Here's how the part is built. I have some questions about the finished solid (model axes, mm). A direction names the side the tool comes from. Coordinates: 2 decimals unless noted, no trailing zeros. Order: outer loops, then holes, each group sorted by start corner. A loop starts at its lowest first (then second) coordinate and runs counter-clockwise, first axis right, second up.
```python
from build123d import *

# Parameters (mm, degrees)
SKETCH2_W           = 21.1
SKETCH2_H           = 50.65
SKETCH2_R           = 5.475
BOSS_EXTRUDE1_DEPTH = 7.5
SKETCH3_W           = 3.15
SKETCH3_H           = 10.4
CUT_EXTRUDE1_DEPTH  = 53.277863384
FILLET1_R           = 0.5
SKETCH4_W           = 11.1
SKETCH4_H           = 21
CUT_EXTRUDE3_DEPTH  = 13
SKETCH6_W           = 11.1
SKETCH6_H           = 18.940672382
CUT_EXTRUDE4_DEPTH  = 13
SKETCH7_W           = 11.1
SKETCH7_H           = 5
CUT_EXTRUDE5_DEPTH  = 1
SKETCH8_W           = 9
SKETCH8_H           = 3
CUT_EXTRUDE6_DEPTH  = 9.8


with BuildPart() as part:
    # Sketch2 → Boss-Extrude1 (new, symmetric)
    with BuildSketch(Plane.XY):
        with Locations((0, 6.8)):
            Rectangle(SKETCH2_W, SKETCH2_H)
        with Locations((0, 6.8)):
            Circle(SKETCH2_R, mode=Mode.SUBTRACT)
    extrude(amount=BOSS_EXTRUDE1_DEPTH, both=True)

    # Sketch3 → Cut-Extrude1 (cut, symmetric)
    with BuildSketch(Plane(origin=(0, 32.125, 0), x_dir=(1, 0, 0), z_dir=(0, 1, 0))):
        with Locations((-8.975, 0)):
            Rectangle(SKETCH3_W, SKETCH3_H)
    cut_extrude1 = extrude(amount=CUT_EXTRUDE1_DEPTH, both=True, mode=Mode.SUBTRACT)

    # Mirror1: Cut-Extrude1 across plane
    add(cut_extrude1.mirror(Plane(origin=(0, 0, 0), x_dir=(0, 0, 1), z_dir=(1, 0, 0))), mode=Mode.SUBTRACT)

    # Fillet1
    fillet1_edges = [part.edges().sort_by_distance(p)[0] for p in [
        (-7.4, 6.8, -5.2),
        (-7.4, 6.8, 5.2),
        (7.4, 6.8, 5.2),
        (7.4, 6.8, -5.2),
    ]]
    fillet(fillet1_edges, radius=FILLET1_R)

    # Sketch4 → Cut-Extrude3 (cut)
    with BuildSketch(Plane(origin=(0, 0, -7.5), x_dir=(-1, 0, 0), z_dir=(0, 0, -1))):
        with Locations((0, 11.825)):
            Rectangle(SKETCH4_W, SKETCH4_H)
    extrude(amount=-CUT_EXTRUDE3_DEPTH, mode=Mode.SUBTRACT)

    # Sketch6 → Cut-Extrude4 (cut)
    with BuildSketch(Plane(origin=(0, 0, -7.5), x_dir=(-1, 0, 0), z_dir=(0, 0, -1))):
        with Locations((0, -10.645336191)):
            Rectangle(SKETCH6_W, SKETCH6_H)
    extrude(amount=-CUT_EXTRUDE4_DEPTH, mode=Mode.SUBTRACT)

    # Sketch7 → Cut-Extrude5 (cut)
    with BuildSketch(Plane(origin=(0, 0, 5.5), x_dir=(-1, 0, 0), z_dir=(0, 0, -1))):
        with Locations((0, 19.825)):
            Rectangle(SKETCH7_W, SKETCH7_H)
    extrude(amount=-CUT_EXTRUDE5_DEPTH, mode=Mode.SUBTRACT)

    # Sketch8 → Cut-Extrude6 (cut)
    with BuildSketch(Plane(origin=(0, 32.125, 0), x_dir=(1, 0, 0), z_dir=(0, 1, 0))):
        with Locations((0, 4.5)):
            Rectangle(SKETCH8_W, SKETCH8_H)
    extrude(amount=-CUT_EXTRUDE6_DEPTH, mode=Mode.SUBTRACT)


solid = part.part
```
Q1. I need wall thicknesses on L1, parallel to Y at x = 4, z = 4 (3 decimals); L2, parallel to X at y = 6.8, z = 6.3 (3 decimals); L3, parallel to Y at x = 0, z = 7.05 (3 decimals). Which ranges of each line are inside material? Lowest first, please.
Q2. We'd pull the mould along Z, two halves only. Please class faces 5 (the flat face through (10.55, 6, 6)), 6 (the flat face through (-7, 13, -7.5)), 7 (the flat face through (7.4, 7, 0)), 8 (the flat face through (-9, 7, 5.2)): pulls with the +Z half, pulls with the -Z half, needs draft (parallel to the pull), parting line crosses it, or undercut.
Q3. If we section it at B-B on z = -1.25: Write out the boundary of the cut face in (x, y) (3 decimals).
Q4. For faces 1 (the flat face through (0, -1.175, -1)), 2 (the flat face through (-7.4, 7, 0)), 3 (the flat face through (5.55, 12, -1)), 4 (the flat face through (-4.5, 27, -4)), which set-ups out of +Z, -Z, +X, -X, +Y, -Y let a thin tool reach every point of the face, with its end or its side?
Q5. Will these pins go through, and if not, where does the flat tip stop? pin 1 (7.5 mm diameter, centred on y = -5.5, z = -0.5, fed in from +X); pin 2 (2 mm diameter, centred on y = 13.5, z = -3.5, fed in from -X); pin 3 (4 mm diameter, centred on x = -1.5, y = 19, fed in from -Z).
Q6. If we section it at C-C on x = -3: Write out the boundary of the cut face in (y, z) (3 decimals).
Q7. If we section it at A-A on y = 6.8: Write out the boundary of the cut face in (x, z) (3 decimals).
Q8. If we section it at D-D on y = 18: Write out the boundary of the cut face in (x, z).
Reply:
1. L1: y = -1.175 to 1.325, 22.325 to 32.125
1. L2: x = -10.55 to -5.475, 5.475 to 10.55
1. L3: y = -18.525 to 1.325, 12.275 to 32.125
2. face 5: needs draft
2. face 6: pulls with the -Z half
2. face 7: undercut
2. face 8: undercut
3. outline: (-7.4, -18.525) - (-5.55, -18.525) - (-5.55, -1.175) - (5.55, -1.175) - (5.55, -18.525) - (7.4, -18.525) - (7.4, 32.125) - (-7.4, 32.125) - close; hole (-5.55, 1.325) - (5.55, 1.325) - (5.55, 22.325) - (-5.55, 22.325) - close
4. face 1: -Z, -Y
4. face 2: -X, +Y, -Y
4. face 3: -Z
4. face 4: +Y
5. pin 1: stops at x = 7.4
5. pin 2: stops at x = -7.4
5. pin 3: stops at z = 5.5
6. outline: (-18.525, 5.5) - (-1.175, 5.5) - (-1.175, -7.5) - (1.325, -7.5) - (1.325, 5.5) - (2.22, 5.5) - (2.22, 7.5) - (-18.525, 7.5) - close; (11.38, 5.5) - (17.325, 5.5) - (17.325, 6.5) - (22.325, 6.5) - (22.325, -3) - (32.125, -3) - (32.125, 7.5) - (11.38, 7.5) - close; (22.325, -7.5) - (32.125, -7.5) - (32.125, -6) - (22.325, -6) - close
7. outline: (-10.55, -7.5) - (-5.55, -7.5) - (-5.55, 5.5) - (-5.475, 5.5) - (-5.475, 7.5) - (-10.55, 7.5) - (-10.55, 5.2) - (-7.9, 5.2) arc R0.5 cw to (-7.4, 4.7) - (-7.4, -4.7) arc R0.5 cw to (-7.9, -5.2) - (-10.55, -5.2) - close; (5.475, 5.5) - (5.55, 5.5) - (5.55, -7.5) - (10.55, -7.5) - (10.55, -5.2) - (7.9, -5.2) arc R0.5 cw to (7.4, -4.7) - (7.4, 4.7) arc R0.5 cw to (7.9, 5.2) - (10.55, 5.2) - (10.55, 7.5) - (5.475, 7.5) - close
8. outline: (-10.55, -7.5) - (-5.55, -7.5) - (-5.55, 6.5) - (5.55, 6.5) - (5.55, -7.5) - (10.55, -7.5) - (10.55, -5.2) - (7.9, -5.2) arc R0.5 cw to (7.4, -4.7) - (7.4, 4.7) arc R0.5 cw to (7.9, 5.2) - (10.55, 5.2) - (10.55, 7.5) - (-10.55, 7.5) - (-10.55, 5.2) - (-7.9, 5.2) arc R0.5 cw to (-7.4, 4.7) - (-7.4, -4.7) arc R0.5 cw to (-7.9, -5.2) - (-10.55, -5.2) - close
